The figure shows three views and two pictorial views of one solid part (mm, origin at its lowest corner). Answer the questions. A direction names the side the tool comes from. Round coordinates to 2 decimals unless told otherwise and drop trailing zeros. Write each loop counter-clockwise with the first axis right and the second up, starting at its lowest first coordinate (ties: lowest second). Pieces come first, ordered by that corner, then holes. Notation, with made-up numbers: (41, -37) - (86, -37) arc R30 ccw to (86, -11) - close; hole circle Ø9 at (-9, 7). An arc over 180 degrees is marked (long way). Answer as CSV lines item,"result". Start each with the question number.
Item 1: A cutting plane is placed at A-A on y = 6.5. Determine the outline of the cut face in (x, z), and give its area (3 significant figures).
Item 2: A cutting plane is placed at C-C on z = 1.5. Determine the outline of the cut face in (x, y).
Item 3: A cutting plane is placed at D-D on x = 30. Determine the outline of the cut face in (y, z), and give its area (3 significant figures).
Item 4: A flat-ended cylindrical pin translates along its axis: pin 1 (1 mm diameter, centred on x = 5.5, z = 0.5, fed in from -Y). Find the tip coordinate at first contact, or state that the pin passes through.
Item 5: Straight lines are drawn through the part: line 1 along Y through (x, z) = (31.5, 0.85); line 2 along X through (y, z) = (8.75, 1.15); line 3 along Z through (x, y) = (30, 1.4). For each, find the intervals that lie inside material, in ascending order. Write a range as [from, to].
Item 6: Which of the six approach directions +Z, -Z, +X, -X, +Y, -Y give full straight-line access (tool end or side, diameter ignored) to the marked faces 1 and 2?
Item 7: For a pull along X with two mould halves and no side action, classify the marked faces 3, 4 and 5 as pulls with the +X half, pulls with the -X half, needs draft (parallel to the pull), parting line crosses it, or undercut.
Item 8: A cutting plane is placed at B-B on x = 45.5. Determine the outline of the cut face in (y, z), and give its area (3 significant figures).
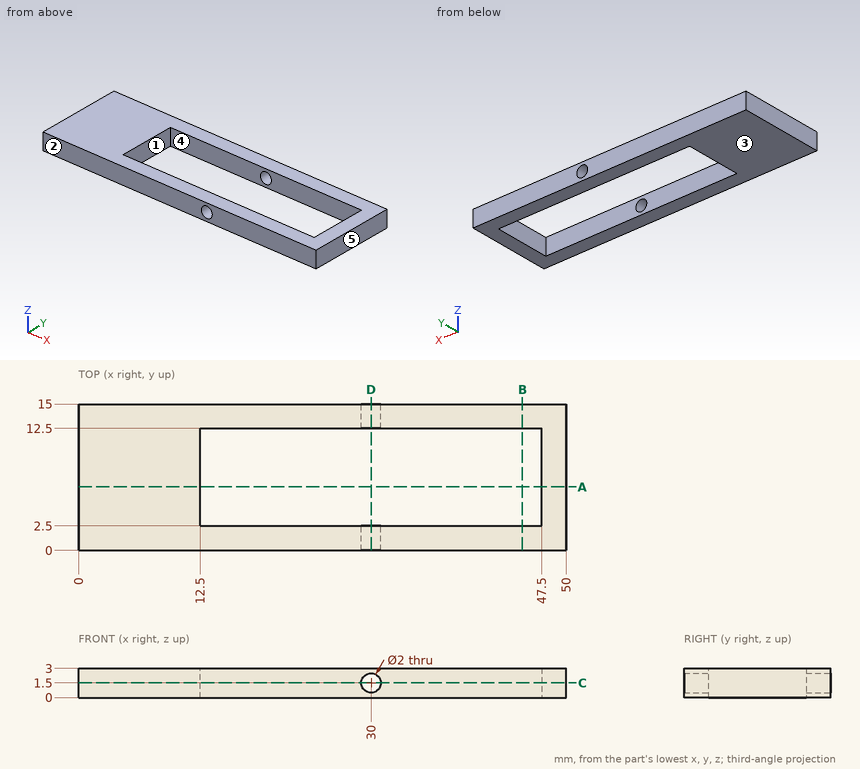
Geometry says:
1,outline,"(0, 0) - (12.5, 0) - (12.5, 3) - (0, 3) - close; (47.5, 0) - (50, 0) - (50, 3) - (47.5, 3) - close"
1,area,"45.0 mm^2"
2,outline,"(0, 0) - (29, 0) - (29, 2.5) - (12.5, 2.5) - (12.5, 12.5) - (29, 12.5) - (29, 15) - (0, 15) - close; (31, 0) - (50, 0) - (50, 15) - (31, 15) - (31, 12.5) - (47.5, 12.5) - (47.5, 2.5) - (31, 2.5) - close"
3,outline,"(0, 0) - (2.5, 0) - (2.5, 0.5) - (0, 0.5) - close; (0, 2.5) - (2.5, 2.5) - (2.5, 3) - (0, 3) - close; (12.5, 0) - (15, 0) - (15, 0.5) - (12.5, 0.5) - close; (12.5, 2.5) - (15, 2.5) - (15, 3) - (12.5, 3) - close"
3,area,"5.00 mm^2"
4,pin 1,"stops at y = 0"
5,line 1,"y = [0, 2.5], [12.5, 15]"
5,line 2,"x = [0, 12.5], [47.5, 50]"
5,line 3,"z = [0, 0.5], [2.5, 3]"
6,face 1,"+Z, -Z"
6,face 2,"+Z, -Z, +X, -X, -Y"
7,face 3,"needs draft"
7,face 4,"undercut"
7,face 5,"pulls with the +X half"
8,outline,"(0, 0) - (2.5, 0) - (2.5, 3) - (0, 3) - close; (12.5, 0) - (15, 0) - (15, 3) - (12.5, 3) - close"
8,area,"15.0 mm^2"
